Can you work these out from the model? Positions are in its coordinate system, mm. A direction names the side the tool comes from. Give positions to 0.01 mm unless a question says otherwise; leave off trailing zeros. Write each loop counter-clockwise with the first axis right and the second up, starting at its lowest first coordinate (ties: lowest second). Pieces come first, ordered by that corner, then holes.
1. Suppose I cut it at C-C (y = 2). Please give me the cut outline in (x, z), and give its area (3 significant figures).
2. Suppose I cut it at A-A (z = 1). Please give me the cut outline in (x, y), and give its area (3 significant figures).
3. Suppose I cut it at B-B (y = -6). Please give me the cut outline in (x, z), and give its area (3 significant figures).
4. If I drill on probe 1 along Z at (x, y) = (-9, 0); probe 2 along Z at (x, y) = (2.25, 14); probe 3 along Y at (x, z) = (-1, -23), over which ranges is the centre line in solid material (lowest first)?
5. Thinking about a two-plate mould opening in Z: for faces 1 (the flat face through (0, 25, -6)), 2 (the cylindrical face through (3.05, -0.96, -22.54)), 3 (the cylindrical face through (-9.718, 4.787, 4.699)), which applies, pulls with the +Z half, pulls with the -Z half, needs draft (parallel to the pull), parting line crosses it, or undercut?
6. Suppose I cut it at D-D (z = -9.5). Please give me the cut outline in (x, y), and give its area (3 significant figures).
7. I'm going to push flat-ended pins straight in: pin 1 (1 mm diameter, centred on x = -3, z = -16, fed in from -Y); pin 2 (5.5 mm diameter, centred on y = 23, z = -10, fed in from -X); pin 3 (6 mm diameter, centred on x = -5.5, z = -22, fed in from +Y). Where does each tip first touch, or does it pass through?
8. On a 3-axis mill with a long thin cutter (end or side, diameter ignored), from which of +Z, -Z, +X, -X, +Y, -Y can I reach the whole of each face in a straight line? I mean faces 4 (the cylindrical face through (9.712, -9.702, -22.465)), 5 (the flat face through (-3.4, 13.99, -9.4)), 6 (the flat face through (-2.4, 2.4, 0)). Say none if no direction works.
```python
from build123d import *
from build123d.topology import SkipClean

# Parameters (mm, degrees)
SKETCH2_R           = 4.200000000000002
SKETCH2_R_2         = 3.2
BOSS_EXTRUDE2_DEPTH = 5
BOSS_EXTRUDE3_START = 20
BOSS_EXTRUDE3_DEPTH = 20
BOSS_EXTRUDE4_START = 6
SKETCH4_R           = 4.200000000000002
BOSS_EXTRUDE4_DEPTH = 6
BOSS_EXTRUDE5_START = 5
SKETCH5_R           = 3.2000000000000006
SKETCH5_R_2         = 4.200000000000001
BOSS_EXTRUDE5_DEPTH = 5
SKETCH6_R           = 4.200000000000002
BOSS_EXTRUDE6_DEPTH = 7.3
FILLET1_R           = 1


with BuildPart() as part:
    # Sketch2 → Boss-Extrude2 (new body)
    with BuildSketch(Plane.XY):
        with BuildLine():
            Line((-10.002730808209856, -10.002730808209863), (9.997269191790144, -10.002730808209856))
            Line((9.997269191790144, -10.002730808209856), (9.997269191790144, 19.99726919179014))
            ThreePointArc((9.997269191790144, 19.99726919179014), (-0.00273080820985792, 29.99726919179014), (-10.002730808209856, 19.997269191790135))
            Line((-10.002730808209856, 19.997269191790135), (-10.002730808209856, -10.002730808209863))
        make_face()
        with Locations((-0.00273080820985608, 19.99726919179014)):
            Circle(SKETCH2_R, mode=Mode.SUBTRACT)
        with Locations((-0.00273080820986128, -0.00273080820986128)):
            Circle(SKETCH2_R_2, mode=Mode.SUBTRACT)
    extrude(amount=BOSS_EXTRUDE2_DEPTH)

    # Sketch3 → Boss-Extrude3 (add)
    with BuildSketch(Plane(origin=(0, 0, 0), x_dir=(-1, 0, 0), z_dir=(0, 0, -1)).offset(BOSS_EXTRUDE3_START)):
        with BuildLine():
            Line((6.9027308082098555, 19.298146779896605), (6.9027308082098555, 27.235362863469167))
            ThreePointArc((6.9027308082098555, 27.235362863469167), (9.195118963634973, 23.934273128796043), (10.002730808209856, 19.99726919179014))
            Line((10.002730808209856, 19.99726919179014), (10.002730808209868, 9.997269191790137))
            Line((10.002730808209868, 9.997269191790137), (-9.997269191790144, 9.997269191790139))
            Line((-9.997269191790144, 9.997269191790139), (-9.997269191790146, 19.99726919179014))
            ThreePointArc((-9.997269191790146, 19.99726919179014), (-9.189657347215263, 23.934273128796043), (-6.897269191790147, 27.235362863469163))
            Line((-6.897269191790147, 27.235362863469163), (-6.897269191790146, 21.118127792576228))
            Line((-6.897269191790146, 21.118127792576228), (-6.897269191790146, 16.01355233438172))
            Line((-6.897269191790146, 16.01355233438172), (0.00273080820985521, 12.029835476973302))
            Line((0.00273080820985521, 12.029835476973302), (6.9027308082098555, 16.013552334381725))
            Line((6.9027308082098555, 16.013552334381725), (6.9027308082098555, 19.298146779896605))
        make_face()
    extrude(amount=-BOSS_EXTRUDE3_DEPTH)

    # Sketch4 → Boss-Extrude4 (add)
    with SkipClean():  # the faces are left unmerged after this step: merging them gives an invalid solid
        with BuildSketch(Plane(origin=(0, 0, 0), x_dir=(-1, 0, 0), z_dir=(0, 0, -1)).offset(BOSS_EXTRUDE4_START)):
            with BuildLine():
                Line((6.9027308082098555, 16.013552334381725), (6.902730808209854, 27.235362863469167))
                ThreePointArc((6.902730808209854, 27.235362863469167), (0.00273080820985225, 29.99726919179014), (-6.897269191790148, 27.235362863469163))
                Line((-6.897269191790148, 27.235362863469163), (-6.897269191790146, 16.01355233438172))
                Line((-6.897269191790146, 16.01355233438172), (0.00273080820985521, 12.029835476973302))
                Line((0.00273080820985521, 12.029835476973302), (6.9027308082098555, 16.013552334381725))
            make_face()
            with Locations((0.00273080820985608, 19.99726919179014)):
                Circle(SKETCH4_R, mode=Mode.SUBTRACT)
        extrude(amount=-BOSS_EXTRUDE4_DEPTH)

    # Sketch5 → Boss-Extrude5 (add)
    # profile 1 of 3: a face of its own
    with SkipClean():  # the faces are left unmerged after this step: merging them gives an invalid solid
        with BuildSketch(Plane(origin=(0, 0, -20), x_dir=(-1, 0, 0), z_dir=(0, 0, -1)).offset(BOSS_EXTRUDE5_START)):
            with BuildLine():
                Line((6.9027308082098555, 16.013552334381725), (0.00273080820985521, 12.029835476973302))
                Line((0.00273080820985521, 12.029835476973302), (-6.897269191790146, 16.01355233438172))
                Line((-6.897269191790146, 16.01355233438172), (-6.897269191790149, 27.235362863469163))
                ThreePointArc((-6.897269191790149, 27.235362863469163), (-9.189657347215263, 23.934273128796043), (-9.997269191790146, 19.99726919179014))
                Line((-9.997269191790146, 19.99726919179014), (-9.997269191790144, 9.997269191790139))
                Line((-9.997269191790144, 9.997269191790139), (10.002730808209868, 9.997269191790137))
                Line((10.002730808209868, 9.997269191790137), (10.002730808209856, 19.99726919179014))
                ThreePointArc((10.002730808209856, 19.99726919179014), (9.195118963634973, 23.934273128796043), (6.9027308082098555, 27.235362863469167))
                Line((6.9027308082098555, 27.235362863469167), (6.9027308082098555, 16.013552334381725))
            make_face()
        # profile 2 of 3: a face of its own
        with BuildSketch(Plane(origin=(0, 0, -20), x_dir=(-1, 0, 0), z_dir=(0, 0, -1)).offset(BOSS_EXTRUDE5_START)):
            Polygon((10.00273080820987, 9.997269191790137), (-9.997269191790144, 9.997269191790139), (-9.997269191790142, -10.002730808209861), (10.002730808209861, -10.002730808209861), align=None)
            with Locations(Location((0.00273080820986128, -0.00273080820986128, 0), (0, 0, 180))):
                Circle(SKETCH5_R, mode=Mode.SUBTRACT)
        # profile 3 of 3: a face of its own
        with BuildSketch(Plane(origin=(0, 0, -20), x_dir=(-1, 0, 0), z_dir=(0, 0, -1)).offset(BOSS_EXTRUDE5_START)):
            with BuildLine():
                ThreePointArc((6.902730808209858, 27.235362863469167), (0.00273080820985499, 29.99726919179014), (-6.897269191790148, 27.235362863469163))
                Line((-6.897269191790149, 27.235362863469163), (-6.897269191790146, 16.01355233438172))
                Line((-6.897269191790146, 16.01355233438172), (0.00273080820985521, 12.029835476973302))
                Line((0.00273080820985516, 12.029835476973302), (6.9027308082098555, 16.013552334381725))
                Line((6.9027308082098555, 16.013552334381725), (6.9027308082098555, 27.235362863469167))
            make_face()
            with Locations((0.00273080820985608, 19.99726919179014)):
                Circle(SKETCH5_R_2, mode=Mode.SUBTRACT)
        extrude(amount=-BOSS_EXTRUDE5_DEPTH)

    # Sketch6 → Boss-Extrude6 (add)
    with SkipClean():  # the faces are left unmerged after this step: merging them gives an invalid solid
        with BuildSketch(Plane.XY.offset(-20)):
            with BuildLine():
                Line((-0.00273080820985521, 12.029835476973302), (6.897269191790146, 16.01355233438172))
                Line((6.897269191790146, 16.01355233438172), (6.897269191790149, 27.235362863469163))
                ThreePointArc((6.897269191790149, 27.235362863469163), (-0.00273080820985102, 29.99726919179014), (-6.9027308082098555, 27.23536286346917))
                Line((-6.9027308082098555, 27.23536286346917), (-6.9027308082098555, 16.013552334381725))
                Line((-6.9027308082098555, 16.013552334381725), (-0.00273080820985521, 12.029835476973302))
            make_face()
            with Locations(Location((-0.00273080820985608, 19.99726919179014, 0), (0, 0, 180))):
                Circle(SKETCH6_R, mode=Mode.SUBTRACT)
        extrude(amount=BOSS_EXTRUDE6_DEPTH)

    # Fillet1
    fillet1_edges = [part.edges().sort_by_distance(p)[0] for p in [
        (9.997269191790144, 4.99726919179014, 5),
        (-0.00273080820985721, 29.99726919179014, 5),
        (-10.002730808209856, 4.997269191790135, 5),
        (-10.002730808209861, -10.002730808209861, -22.5),
        (9.997269191790142, -10.002730808209861, -22.5),
        (-10.002730808209858, 4.997269191790139, -25),
        (-0.00273080820987453, 29.99726919179015, -25),
        (9.997269191790144, 4.997269191790139, -25),
        (9.997269191790144, -10.002730808209856, 2.5),
        (-10.002730808209856, -10.002730808209863, 2.5),
    ]]
    fillet(fillet1_edges, radius=FILLET1_R)


solid = part.part
```
Checks:
1. outline: (-10, -24) arc R1 ccw to (-9, -25) - (-2.5, -25) - (-2.5, -20) - (-10, -20) - close; (-10, 0) - (-2.5, 0) - (-2.5, 5) - (-9, 5) arc R1 ccw to (-10, 4) - close; (2.49, -25) - (9, -25) arc R1 ccw to (10, -24) - (10, -20) - (2.49, -20) - close; (2.49, 0) - (10, 0) - (10, 4) arc R1 ccw to (9, 5) - (2.49, 5) - close
1. area: 149 mm2
2. outline: (-10, -9) arc R1 ccw to (-9, -10) - (9, -10) arc R1 ccw to (10, -9) - (10, 20) arc R10 ccw to (-10, 20) - close; hole circle Ø8.4 at (0, 20); hole circle Ø6.4 at (0, 0)
2. area: 669 mm2
3. outline: (-10, -24) arc R1 ccw to (-9, -25) - (9, -25) arc R1 ccw to (10, -24) - (10, -20) - (-10, -20) - close; (-10, 0) - (10, 0) - (10, 4) arc R1 ccw to (9, 5) - (-9, 5) arc R1 ccw to (-10, 4) - close
3. area: 199 mm2
4. probe 1: z = -25 to -20, 0 to 5
4. probe 2: z = -25 to -12.7, -6 to 5
4. probe 3: y = -10 to -3.04, 3.04 to 15.92, 24.08 to 29.95
5. face 1: undercut
5. face 2: needs draft
5. face 3: pulls with the +Z half
6. outline: (-10, 10) - (10, 10) - (10, 20) arc R10 ccw to (6.9, 27.24) - (6.9, 16.01) - (0, 12.03) - (-6.9, 16.01) - (-6.9, 27.24) arc R10 ccw to (-10, 20) - close
6. area: 149 mm2
7. pin 1: stops at y = 10
7. pin 2: stops at x = -10
7. pin 3: stops at y = 29.68
8. face 4: +Z, -Z, +X, -Y
8. face 5: +Y
8. face 6: +X, -X, -Y
